Verification items for the finished model (mm, model axes). Face numbers are marked on the shaded views. A direction names the side the tool comes from. Round coordinates to 2 decimals unless told otherwise and drop trailing zeros. Order: outer loops, then holes, each group sorted by start corner. A loop starts at its lowest first (then second) coordinate and runs counter-clockwise, first axis right, second up. Notation, with made-up numbers: (-34.5, 1.5) -> (1.5, 1.5) arc R9 cw to (1.5, 9.5) -> close; hole circle Ø8 at (27, -2.5). An arc over 180 degrees is marked (long way). Answer in a Markdown table with one row per item. Add a question column.
```python
from build123d import *

# Parameters (mm, degrees)
ENL_V_MAT_EXTRU_1_DEPTH = 2.2


with BuildPart() as part:
    # Esquisse1 → Révolution1 (revolve)
    with BuildSketch(Plane.XY, mode=Mode.PRIVATE) as r_volution1_sk:
        Polygon((-8.5, 3.7), (-1.25, 3.7), (-1.25, 2.2), (-2.2, 2.2), (-2.2, 0), (-3.9, 0), (-3.9, 2.2), (-8.5, 2.2), align=None)
    revolve(r_volution1_sk.sketch.rotate(Axis((0, 0, 0), (0, 1, 0)), 270), axis=Axis((0, 0, 0), (0, 1, 0)))

    # Esquisse2 → Enlèv. mat.-Extru.1 (cut)
    with BuildSketch(Plane.XZ):
        Polygon((1.274522619, -1.907457896), (1.907457896, -1.274522619), (2.25, -0.447552827), (2.25, 0.447552827), (1.907457896, 1.274522619), (1.274522619, 1.907457896), (0.447552827, 2.25), (-0.447552827, 2.25), (-1.274522619, 1.907457896), (-1.907457896, 1.274522619), (-2.25, 0.447552827), (-2.25, -0.447552827), (-1.907457896, -1.274522619), (-1.274522619, -1.907457896), (-0.447552827, -2.25), (0.447552827, -2.25), align=None)
    extrude(amount=-ENL_V_MAT_EXTRU_1_DEPTH, mode=Mode.SUBTRACT)


solid = part.part
```
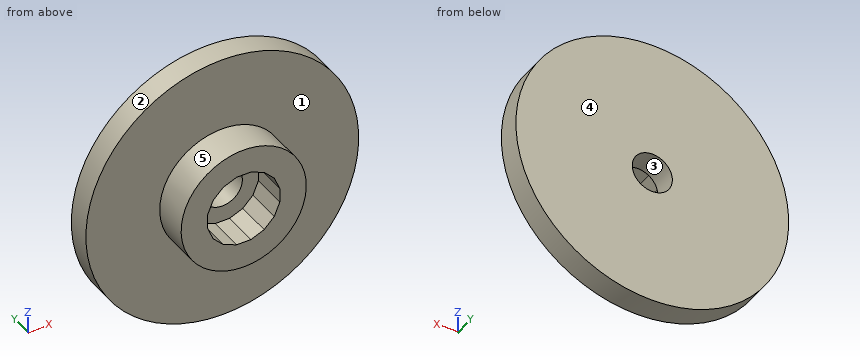
1) Cross-section at D-D, the plane y = 3.2. Record the boundary of the cut face in (x, z).
2) Depth check by flat-ended pin: P1, Ø0.7, axis at y = 1.5, z = 0, coming from the -X side; P2, Ø4, axis at x = 0, z = 0, coming from the +Y side; P3, Ø2, axis at x = -0.5, z = 0.5, coming from the -Y side; P4, Ø0.7, axis at x = 0, y = 1.5, coming from the +Z side. Enter the tip coordinate at first touch or a pass-through.
3) Cross-section at B-B, the plane z = 0. Record the boundary of the cut face in (x, y), and give its area (3 significant figures).
4) Draft check along Z on the marked faces 1, 2 and 3. Enter one of: +Z half, -Z half, draft (parallel to the pull), parting line (faces both ways), or undercut.
5) Cross-section at A-A, the plane x = 0. Record the boundary of the cut face in (y, z), and give its area (3 significant figures).
6) Cross-section at C-C, the plane x = -3. Record the boundary of the cut face in (y, z), and give its area (3 significant figures).
7) Tool access check on the marked faces 4 and 5. Record the directions out of +Z, -Z, +X, -X, +Y, -Y that give a thin tool (end or side, any length) a straight path to the whole face; none if there is none.
8) Thickness scan on L1, parallel to X at y = 2.5, z = 0; L2, parallel to Y at x = -4.5, z = 0.25; L3, parallel to X at y = 1.15, z = 0.75. Record the ranges inside material, lowest first. Write a range as [from, to].
Results below:
| question | item | result |
|---|---|---|
| 1 | outline | circle Ø17 at (0, 0); hole circle Ø2.5 at (0, 0) |
| 2 | P1 | x = -3.9 |
| 2 | P2 | y = 3.7 |
| 2 | P3 | y = 2.2 |
| 2 | P4 | z = 3.9 |
| 3 | outline | (-8.5, 2.2) -> (-3.9, 2.2) -> (-3.9, 0) -> (-2.25, 0) -> (-2.25, 2.2) -> (-1.25, 2.2) -> (-1.25, 3.7) -> (-8.5, 3.7) -> close; (1.25, 2.2) -> (2.25, 2.2) -> (2.25, 0) -> (3.9, 0) -> (3.9, 2.2) -> (8.5, 2.2) -> (8.5, 3.7) -> (1.25, 3.7) -> close |
| 3 | area | 29.0 mm² |
| 4 | face 1 | draft |
| 4 | face 2 | parting line |
| 4 | face 3 | undercut |
| 5 | outline | (0, -3.9) -> (2.2, -3.9) -> (2.2, -8.5) -> (3.7, -8.5) -> (3.7, -1.25) -> (2.2, -1.25) -> (2.2, -2.25) -> (0, -2.25) -> close; (0, 2.25) -> (2.2, 2.25) -> (2.2, 1.25) -> (3.7, 1.25) -> (3.7, 8.5) -> (2.2, 8.5) -> (2.2, 3.9) -> (0, 3.9) -> close |
| 5 | area | 29.0 mm² |
| 6 | outline | (0, -2.49) -> (2.2, -2.49) -> (2.2, -7.95) -> (3.7, -7.95) -> (3.7, 7.95) -> (2.2, 7.95) -> (2.2, 2.49) -> (0, 2.49) -> close |
| 6 | area | 34.8 mm² |
| 7 | face 4 | +Z, -Z, +X, -X, +Y |
| 7 | face 5 | -Y |
| 8 | L1 | [-8.5, -1.25], [1.25, 8.5] |
| 8 | L2 | [2.2, 3.7] |
| 8 | L3 | [-3.83, -2.12], [2.12, 3.83] |
